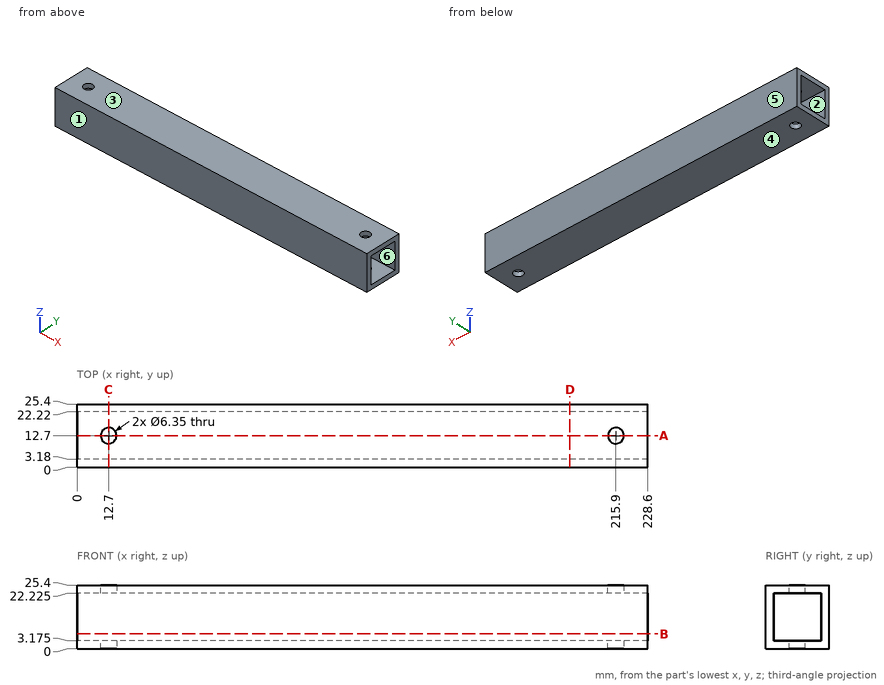
Here's the drawing with two shaded views (mm, measured from the low corner). I have some questions. A direction names the side the tool comes from. Round coordinates to 2 decimals unless told otherwise and drop trailing zeros. Order: outer loops, then holes, each group sorted by start corner. A loop starts at its lowest first (then second) coordinate and runs counter-clockwise, first axis right, second up. Notation, with made-up numbers: (-27.75, 30) -> (-4.75, 30) arc R9 ccw to (-4.75, 46) -> close; hole circle Ø9 at (37, 72.5). An arc over 180 degrees is marked (long way). Write each question's results on one line, items separated by ' | '. Start each with the question number.
Item 1: If we section it at C-C, the plane x = 12.7: Write out the boundary of the cut face in (y, z) (1 decimal), then the cut area to 3 significant figures.
Item 2: Please list where these lines run through material, in increasing order: L1, parallel to Z at x = 86, y = 8.5 (1 decimal); L2, parallel to Y at x = 185, z = 10.75; L3, parallel to Y at x = 12.7, z = 23.8 (1 decimal).
Item 3: Which directions (+Z, -Z, +X, -X, +Y, -Y) give clear straight access to the entire face, cutting with the end or side of a thin tool? Please do the marked faces 1 and 2.
Item 4: If we section it at B-B, the plane z = 6: Write out the boundary of the cut face in (x, y), then the cut area to 3 significant figures.
Item 5: Will this pin go through, and if not, where does the flat tip stop? pin 1 (5 mm diameter, centred on x = 12.7, y = 12.7, fed in from +Z).
Item 6: Thinking about a two-plate mould opening in Z: for the marked faces 3, 4, 5 and 6, which applies, +Z half, -Z half, draft (parallel to the pull), parting line (faces both ways), or undercut?
Item 7: If we section it at D-D, the plane x = 197.5: Write out the boundary of the cut face in (y, z) (1 decimal).
Item 8: If we section it at A-A, the plane y = 12.7: Write out the boundary of the cut face in (x, z) (1 decimal).
Results:
1) outline: (0, 0) -> (9.5, 0) -> (9.5, 3.2) -> (3.2, 3.2) -> (3.2, 22.2) -> (9.5, 22.2) -> (9.5, 25.4) -> (0, 25.4) -> close; (15.9, 0) -> (25.4, 0) -> (25.4, 25.4) -> (15.9, 25.4) -> (15.9, 22.2) -> (22.2, 22.2) -> (22.2, 3.2) -> (15.9, 3.2) -> close | area: 242 mm2
2) L1: z = 0 to 3.2, 22.2 to 25.4 | L2: y = 0 to 3.18, 22.22 to 25.4 | L3: y = 0 to 9.5, 15.9 to 25.4
3) face 1: +Z, -Z, +X, -X, -Y | face 2: +X, -X
4) outline: (0, 0) -> (228.6, 0) -> (228.6, 3.18) -> (0, 3.18) -> close; (0, 22.22) -> (228.6, 22.22) -> (228.6, 25.4) -> (0, 25.4) -> close | area: 1,450 mm2
5) pin 1: passes through
6) face 3: +Z half | face 4: -Z half | face 5: draft | face 6: undercut
7) outline: (0, 0) -> (25.4, 0) -> (25.4, 25.4) -> (0, 25.4) -> close; hole (3.2, 3.2) -> (22.2, 3.2) -> (22.2, 22.2) -> (3.2, 22.2) -> close
8) outline: (0, 0) -> (9.5, 0) -> (9.5, 3.2) -> (0, 3.2) -> close; (0, 22.2) -> (9.5, 22.2) -> (9.5, 25.4) -> (0, 25.4) -> close; (15.9, 0) -> (212.7, 0) -> (212.7, 3.2) -> (15.9, 3.2) -> close; (15.9, 22.2) -> (212.7, 22.2) -> (212.7, 25.4) -> (15.9, 25.4) -> close; (219.1, 0) -> (228.6, 0) -> (228.6, 3.2) -> (219.1, 3.2) -> close; (219.1, 22.2) -> (228.6, 22.2) -> (228.6, 25.4) -> (219.1, 25.4) -> close
